Check sheet for the modelled part. Datum: model origin and axes. Units: mm. A direction names the side the tool comes from. Round coordinates to 2 decimals unless told otherwise and drop trailing zeros. Order: outer loops, then holes, each group sorted by start corner. A loop starts at its lowest first (then second) coordinate and runs counter-clockwise, first axis right, second up.
(1) Mould release check, pull along Y, two halves, no side actions. Record for faces 3 (the flat face through (-3, 4, 9.947)), 4 (the flat face through (-3, -279.4, 0)), 5 (the flat face through (-3, 279.4, 0)), 6 (the flat face through (-3, 4, 12.7)): released by +Y, released by -Y, zero draft, split by the parting line, or undercut.
(2) Thickness scan on probe 1 along X at (y, z) = (254, 11.1) (3 decimals); probe 2 along Y at (x, z) = (-222.25, 11.55); probe 3 along X at (y, z) = (152, -3.5) (3 decimals). Record the ranges inside material, lowest first.
(3) Depth check by flat-ended pin: pin 1 (6.5 mm diameter, centred on x = -151.61, y = 225.42, fed in from +Z). Enter the tip coordinate at first touch or a pass-through.
(4) Sectioned sample at A-A, the plane z = -5.5. Enter the section's corners in (x, y) (3 decimals).
(5) Tool access check on faces 1 (the flat face through (238.125, -4, 0)), 2 (the flat face through (-3, 276.647, -1)). Record the directions out of +Z, -Z, +X, -X, +Y, -Y that give a thin tool (end or side, any length) a straight path to the whole face; none if there is none.
(6) Sectioned sample at C-C, the plane y = -182. Enter the section's corners in (x, z) (3 decimals), and give its area (3 significant figures).
(7) Sectioned sample at B-B, the plane x = 65. Enter the section's corners in (y, z), and give its area (3 significant figures).
```python
from build123d import *

# Parameters (mm, degrees)
F0_W     = 476.25
F0_H     = 558.8
F1_DEPTH = 12.7
F2_T     = -2.75336
F3_R     = 2.579688
F4_DEPTH = 25.401


with BuildPart() as f1:
    # F0 (on Top) → F1 (new body, symmetric)
    with BuildSketch(Plane.XY):
        Rectangle(F0_W, F0_H)
    extrude(amount=F1_DEPTH, both=True)

    # F2
    f2_openings = [f1.faces().sort_by_distance(p)[0] for p in [
        (0, 0, -12.7),
    ]]
    offset(amount=F2_T, openings=f2_openings)

    # F3 (on face) → F4 (cut, through all)
    with BuildSketch(Plane.XY.offset(12.7)):
        with Locations((-151.60625, 225.425)):
            Circle(F3_R)
        with Locations((151.60625, 225.425)):
            Circle(F3_R)
        with Locations((151.60625, -198.4375)):
            Circle(F3_R)
        with Locations((-151.60625, -198.4375)):
            Circle(F3_R)
        with Locations((-222.25, -254)):
            Circle(F3_R)
        with Locations((-222.25, 254)):
            Circle(F3_R)
        with Locations((222.25, -254)):
            Circle(F3_R)
        with Locations((222.25, 254)):
            Circle(F3_R)
        with Locations((-222.25, 0)):
            Circle(F3_R)
        with Locations((222.25, 0)):
            Circle(F3_R)
    extrude(amount=-F4_DEPTH, mode=Mode.SUBTRACT)


solid = f1.part
```
Derived:
1. face 3: undercut
1. face 4: released by -Y
1. face 5: released by +Y
1. face 6: zero draft
2. probe 1: x = -238.125 to -224.83, -219.67 to 219.67, 224.83 to 238.125
2. probe 2: y = -279.4 to -256.58, -251.42 to -2.58, 2.58 to 251.42, 256.58 to 279.4
2. probe 3: x = -238.125 to -235.372, 235.372 to 238.125
3. pin 1: stops at z = 12.7
4. outline: (-238.125, -279.4) - (238.125, -279.4) - (238.125, 279.4) - (-238.125, 279.4) - close; hole (-235.372, -276.647) - (235.372, -276.647) - (235.372, 276.647) - (-235.372, 276.647) - close
5. face 1: +Z, -Z, +X, +Y, -Y
5. face 2: -Z
6. outline: (-238.125, -12.7) - (-235.372, -12.7) - (-235.372, 9.947) - (235.372, 9.947) - (235.372, -12.7) - (238.125, -12.7) - (238.125, 12.7) - (-238.125, 12.7) - close
6. area: 1,440 mm2
7. outline: (-279.4, -12.7) - (-276.65, -12.7) - (-276.65, 9.95) - (276.65, 9.95) - (276.65, -12.7) - (279.4, -12.7) - (279.4, 12.7) - (-279.4, 12.7) - close
7. area: 1,660 mm2
